Autodesk Fusion 360 part; units mm, degrees
sketch "Sketch1" plane through (0, 0, 0) normal (0, 0, 1) x (1, 0, 0) in component "Component"
  circle A0 centre (0, 0) radius 1.55
  circle A1 centre (0, 0) radius 6.45
  line L0 (-3.8891, 2.4042) -> (-5.2425, 3.7575)
  line L1 (-3.1466, 3.1466) -> (-3.8891, 2.4042)
  line L2 (-3.1466, 3.1466) -> (-2.4042, 3.8891)
  line L3 (-2.4042, 3.8891) -> (-3.7575, 5.2425)
  line L4 (-2.4042, -3.8891) -> (-3.7575, -5.2425)
  line L5 (-3.1466, -3.1466) -> (-2.4042, -3.8891)
  line L6 (-3.1466, -3.1466) -> (-3.8891, -2.4042)
  line L7 (-3.8891, -2.4042) -> (-5.2425, -3.7575)
  line L8 (3.8891, -2.4042) -> (5.2425, -3.7575)
  line L9 (3.1466, -3.1466) -> (3.8891, -2.4042)
  line L10 (3.1466, -3.1466) -> (2.4042, -3.8891)
  line L11 (2.4042, -3.8891) -> (3.7575, -5.2425)
  line L12 (2.4042, 3.8891) -> (3.7575, 5.2425)
  line L13 (3.1466, 3.1466) -> (2.4042, 3.8891)
  line L14 (3.1466, 3.1466) -> (3.8891, 2.4042)
  line L15 (3.8891, 2.4042) -> (5.2425, 3.7575)
  circle A2 centre (0, 0) radius 2
  line L16 (-1.9799, 3.8891) -> (-3.5052, 5.4144)
  line L17 (-2.9345, 2.9345) -> (-1.9799, 3.8891)
  line L18 (-2.9345, 2.9345) -> (-3.8891, 1.9799)
  line L19 (-3.8891, 1.9799) -> (-5.4144, 3.5052)
  line L20 (-3.8891, -1.9799) -> (-5.4144, -3.5052)
  line L21 (-2.9345, -2.9345) -> (-3.8891, -1.9799)
  line L22 (-2.9345, -2.9345) -> (-1.9799, -3.8891)
  line L23 (-1.9799, -3.8891) -> (-3.5052, -5.4144)
  line L24 (1.9799, -3.8891) -> (3.5052, -5.4144)
  line L25 (2.9345, -2.9345) -> (1.9799, -3.8891)
  line L26 (2.9345, -2.9345) -> (3.8891, -1.9799)
  line L27 (3.8891, -1.9799) -> (5.4144, -3.5052)
  line L28 (3.8891, 1.9799) -> (5.4144, 3.5052)
  line L29 (2.9345, 2.9345) -> (3.8891, 1.9799)
  line L30 (2.9345, 2.9345) -> (1.9799, 3.8891)
  line L31 (1.9799, 3.8891) -> (3.5052, 5.4144)
  dimension "d1" = 3.1
  dimension "d2" = 12.9
  dimension "d13" = 360
extrude "Extrude1" add sketch "Sketch1" along normal blind 3 contours A1 L16 L17 L18 L19 L20 L21 L22 L23 L24 L25 L26 L27 L28 L29 L30 L31 | A1 L12 L13 L14 L15 L28 L29 L30 L31 | A1 L8 L9 L10 L11 L24 L25 L26 L27 | A1 L0 L1 L2 L3 L16 L17 L18 L19 | A1 L4 L5 L6 L7 L20 L21 L22 L23 | A2 in component "Component"
extrude "Extrude2" cut 1 faces at (0.1484, 4.7376, 0) along direction (0, 0, 1) blind 2 in component "Component"
extrude "Extrude3" add sketch "Sketch1" along normal blind 2 contours A1 L12 L13 L14 L15 L28 L29 L30 L31 | A1 L8 L9 L10 L11 L24 L25 L26 L27 | A1 L0 L1 L2 L3 L16 L17 L18 L19 | A1 L4 L5 L6 L7 L20 L21 L22 L23 | A2 in component "Component"
extrude "Extrude4" add sketch "Sketch1" along normal blind 1 contours A1 L16 L17 L18 L19 L20 L21 L22 L23 L24 L25 L26 L27 L28 L29 L30 L31 in component "Component"
extrude "Extrude5" cut sketch "Sketch1" along normal blind 5 contours A2 in component "Component"
extrude "Extrude6" add sketch "Sketch1" along normal blind 3.2 contours A2 in component "Component"
extrude "Extrude7" add sketch "Sketch1" against normal blind 0.2 contours A2 in component "Component"
component "Component" placed x (1, 0, 0) y (0, 1, 0) z (0, 0, 1) at (0, 0, 0)
Geometry: final body of the model. Coordinates: model frame, mm. A direction names the side the tool comes from. Coordinates: 2 decimals unless noted, no trailing zeros. Loops run counter-clockwise (first coordinate to the right, second up) from the corner with the lowest first, then second, coordinate; pieces in that order, holes last. Notation, with made-up numbers: (76.5, -23) -> (85.5, -23) arc R11 ccw to (85.5, -7) -> close; hole circle Ø1 at (11.25, 78.5). An arc over 180 degrees is marked (long way). Use a Markdown table: item, result. Add a question column.
(1) Mould query, pull axis Y, two halves, no side actions, for faces 6 (the cylindrical face through (0.715, 1.375, 1.476)), 7 (the flat face through (-2, -1, 2)), 8 (the flat face through (1, 2, 3)), 9 (the flat face through (4.556, -3.071, 1.479)). Classes: pulls with the +Y half, pulls with the -Y half, needs draft (parallel to the pull), parting line crosses it, or undercut.
(2) Pin query (flat end, axial travel): pin 1 Ø3 at (x, y) = (-3.5, -0.5) entering from +Z; pin 2 Ø1.9 at (x, y) = (0, 0) entering from -Z. Return the tip coordinate at first contact, or that it passes through.
(3) Section query A-A, the plane x = 0. Return loops of the section in (y, z), plus the area to 3 significant figures.
(4) Section query C-C, the plane y = 2.75. Return loops of the section in (x, z).
(5) Line query: line 1 along Y through (x, z) = (0, 2.5); line 2 along Z through (x, y) = (5, 1.5); line 3 along X through (y, z) = (3.25, 0.7). Output: solid intervals per line, ascending.
(6) Access query for faces 1 (the flat face through (-2.95, 2.92, 1.49)), 2 (the flat face through (3.071, 4.556, 1.479)), 3 (the flat face through (-4.556, -3.071, 1.479)), 4 (the flat face through (-3.071, 4.556, 1.479)), 5 (the flat face through (4.64, 2.73, 1.49)). Directions: +Z, -Z, +X, -X, +Y, -Y. A direction counts if a zero-diameter tool reaches every point of the face in a straight line with its end or side. Return the directions, or none.
Answer:
| question | item | result |
|---|---|---|
| 1 | face 6 | undercut |
| 1 | face 7 | undercut |
| 1 | face 8 | needs draft |
| 1 | face 9 | pulls with the -Y half |
| 2 | pin 1 | stops at z = 3 |
| 2 | pin 2 | passes through |
| 3 | outline | (-6.45, 0) -> (-2, 0) -> (-2, -0.2) -> (-1.55, -0.2) -> (-1.55, 3.2) -> (-2, 3.2) -> (-2, 3) -> (-6.45, 3) -> (-6.45, 2) -> (-2, 2) -> (-2, 1) -> (-6.45, 1) -> close; (1.55, -0.2) -> (2, -0.2) -> (2, 0) -> (6.45, 0) -> (6.45, 1) -> (2, 1) -> (2, 2) -> (6.45, 2) -> (6.45, 3) -> (2, 3) -> (2, 3.2) -> (1.55, 3.2) -> close |
| 3 | area | 20.9 mm^2 |
| 4 | outline | (-5.83, 0) -> (-4.23, 0) -> (-4.23, 3) -> (-5.83, 3) -> (-5.83, 2) -> (-4.66, 2) -> (-4.66, 1) -> (-5.83, 1) -> close; (-3.54, 0) -> (3.54, 0) -> (3.54, 3) -> (-3.54, 3) -> close; (4.23, 0) -> (5.83, 0) -> (5.83, 1) -> (4.66, 1) -> (4.66, 2) -> (5.83, 2) -> (5.83, 3) -> (4.23, 3) -> close; hole (-3.12, 1) -> (3.12, 1) -> (3.12, 2) -> (-3.12, 2) -> close |
| 5 | line 1 | y = -6.45 to -1.55, 1.55 to 6.45 |
| 5 | line 2 | z = 0 to 1, 2 to 3 |
| 5 | line 3 | x = -5.57 to -4.73, -3.04 to 3.04, 4.73 to 5.57 |
| 6 | face 1 | none |
| 6 | face 2 | +Z, -Z, +X |
| 6 | face 3 | +Z, -Z, -Y |
| 6 | face 4 | +Z, -Z, -X |
| 6 | face 5 | +X |
